```python
from build123d import *

# Parameters (mm, degrees)
SKETCH_1_R          = 30
EXTRUDE_2_DEPTH     = 6
SKETCH_6_W          = 8
SKETCH_6_H          = 8
CUT_EXTRUDE_2_DEPTH = 45.09081537


with BuildPart() as part:
    # 草图1 → 凸台-拉伸2 (new, symmetric)
    with BuildSketch(Plane.XY):
        Circle(SKETCH_1_R)
    extrude(amount=EXTRUDE_2_DEPTH, both=True)

    # 草图6 → 切除-拉伸2 (cut, through all)
    with BuildSketch(Plane.XY.offset(6)):
        with BuildLine():
            Line((-0.6, 28.993792439), (-0.6, 5))
            Line((-0.6, 5), (-5, 5))
            Line((-5, 5), (-5, 0.6))
            Line((-5, 0.6), (-28.993792439, 0.6))
            ThreePointArc((-28.993792439, 0.6), (-20.506096654, 20.506096654), (-0.6, 28.993792439))
        make_face()
        with BuildLine():
            Line((-28.993792439, -0.6), (-5, -0.6))
            Line((-5, -0.6), (-5, -5))
            Line((-5, -5), (-0.6, -5))
            Line((-0.6, -5), (-0.6, -28.993792439))
            ThreePointArc((-0.6, -28.993792439), (-20.506096654, -20.506096654), (-28.993792439, -0.6))
        make_face()
        with BuildLine():
            Line((0.6, 28.993792439), (0.6, 5))
            Line((0.6, 5), (5, 5))
            Line((5, 5), (5, 0.6))
            Line((5, 0.6), (28.993792439, 0.6))
            ThreePointArc((28.993792439, 0.6), (20.506096654, 20.506096654), (0.6, 28.993792439))
        make_face()
        with BuildLine():
            Line((5, -0.6), (28.993792439, -0.6))
            ThreePointArc((28.993792439, -0.6), (20.506096654, -20.506096654), (0.6, -28.993792439))
            Line((0.6, -28.993792439), (0.6, -5))
            Line((0.6, -5), (5, -5))
            Line((5, -5), (5, -0.6))
        make_face()
        Rectangle(SKETCH_6_W, SKETCH_6_H)
    extrude(amount=-CUT_EXTRUDE_2_DEPTH, mode=Mode.SUBTRACT)


solid = part.part
```
CAD build for the part. Positions are in the model's coordinates, mm. A direction names the side the tool comes from. Coordinates: 2 decimals unless noted, no trailing zeros. Order: outer loops, then holes, each group sorted by start corner. A loop starts at its lowest first (then second) coordinate and runs counter-clockwise, first axis right, second up. Notation, with made-up numbers: (-18, 72) - (4, 72) arc R16 ccw to (4, 102) - close; hole circle Ø5 at (59.5, -5.75). An arc over 180 degrees is marked (long way). Use a Markdown table: item, result. Add a question column.
(1) Flat gauge pins, fed straight in: pin 1 (3 mm diameter, centred on x = -19, z = 0.5, fed in from -Y); pin 2 (2 mm diameter, centred on y = 6.5, z = 2, fed in from +X); pin 3 (6 mm diameter, centred on x = -15, z = 2, fed in from -Y). Where does each tip first touch, or does it go through?
(2) Saw through at C-C (x = -17.5). Give the cut face in (y, z).
(3) Pull direction X, two halves, no side cores. Call faces 1 (the face through (-29.97, 1.32, 0.08)), 2 (the face through (-5, 0, -6)), 3 (the face through (0.6, -17, 0)): +X half, -X half, draft (parallel to the pull), parting line (faces both ways), or undercut.
(4) Saw through at A-A (z = 4). Give the cut face in (x, y).
(5) Which spindle directions (+Z, -Z, +X, -X, +Y, -Y) get a long thin tool onto all of the face, cutting with end or side? Do faces 4 (the face through (5, 3, 0)), 5 (the face through (-5, 0, 6)). Say none if no direction does.
(6) Saw through at B-B (y = 2.5). Give the cut face in (x, z).
(7) Drill centre lines: line 1 along X through (y, z) = (14.5, 0); line 2 along X through (y, z) = (15.5, -2.25); line 3 along Y through (x, z) = (-2, 4.25). Where is each one in solid material? Low to high. Write a range as [from, to].
(8) Saw through at D-D (y = 17). Give the cut face in (x, z).
Solved:
| question | item | result |
|---|---|---|
| 1 | pin 1 | stops at y = -24.37 |
| 1 | pin 2 | stops at x = 29.49 |
| 1 | pin 3 | stops at y = -27.5 |
| 2 | outline | (-24.37, -6) - (-23.12, -6) - (-23.12, 6) - (-24.37, 6) - close; (-0.6, -6) - (0.6, -6) - (0.6, 6) - (-0.6, 6) - close; (23.12, -6) - (24.37, -6) - (24.37, 6) - (23.12, 6) - close |
| 3 | face 1 | parting line |
| 3 | face 2 | draft |
| 3 | face 3 | undercut |
| 4 | outline | circle Ø60 at (0, 0); hole (-28.99, -0.6) arc R29 ccw to (-0.6, -28.99) - (-0.6, -5) - (-5, -5) - (-5, -0.6) - close; hole (-28.99, 0.6) - (-5, 0.6) - (-5, 5) - (-0.6, 5) - (-0.6, 28.99) arc R29 ccw to start; hole (-4, -4) - (4, -4) - (4, 4) - (-4, 4) - close; hole (0.6, -28.99) arc R29 ccw to (28.99, -0.6) - (5, -0.6) - (5, -5) - (0.6, -5) - close; hole (0.6, 5) - (5, 5) - (5, 0.6) - (28.99, 0.6) arc R29 ccw to (0.6, 28.99) - close |
| 5 | face 4 | +Z, -Z |
| 5 | face 5 | +Z, +X, -X, +Y, -Y |
| 6 | outline | (-29.9, -6) - (-28.89, -6) - (-28.89, 6) - (-29.9, 6) - close; (-5, -6) - (-4, -6) - (-4, 6) - (-5, 6) - close; (4, -6) - (5, -6) - (5, 6) - (4, 6) - close; (28.89, -6) - (29.9, -6) - (29.9, 6) - (28.89, 6) - close |
| 7 | line 1 | x = [-26.26, -25.11], [-0.6, 0.6], [25.11, 26.26] |
| 7 | line 2 | x = [-25.69, -24.51], [-0.6, 0.6], [24.51, 25.69] |
| 7 | line 3 | y = [-29.93, -28.93], [-5, -4], [4, 5], [28.93, 29.93] |
| 8 | outline | (-24.72, -6) - (-23.49, -6) - (-23.49, 6) - (-24.72, 6) - close; (-0.6, -6) - (0.6, -6) - (0.6, 6) - (-0.6, 6) - close; (23.49, -6) - (24.72, -6) - (24.72, 6) - (23.49, 6) - close |
